The listing builds one solid part. Answer for the finished solid, in the listing's coordinates (mm). Face numbers are marked on the shaded views. A direction names the side the tool comes from. Coordinates: 2 decimals unless noted, no trailing zeros. Write each loop counter-clockwise with the first axis right and the second up, starting at its lowest first coordinate (ties: lowest second). Pieces come first, ordered by that corner, then holes.
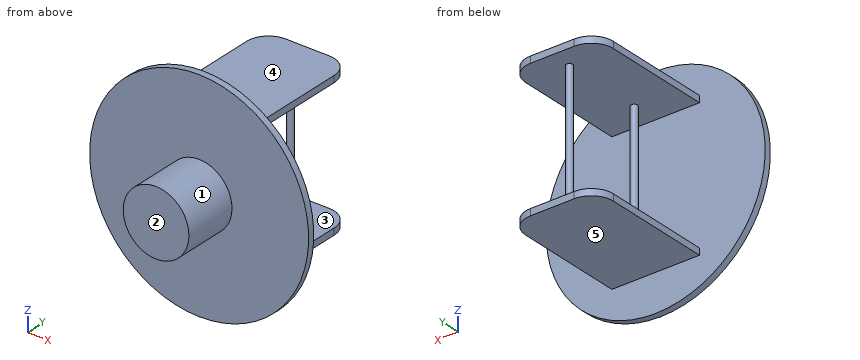
from build123d import *

# Parameters (mm, degrees)
SKETCH1_R           = 50
BOSS_EXTRUDE1_DEPTH = 3
SKETCH2_R           = 15
BOSS_EXTRUDE2_DEPTH = 25
SKETCH3_W           = 40
SKETCH3_H           = 3
BOSS_EXTRUDE3_DEPTH = 60
SKETCH4_R           = 1.5
BOSS_EXTRUDE4_DEPTH = 63
FILLET1_R           = 10


with BuildPart() as part:
    # Sketch1 → Boss-Extrude1 (new body)
    with BuildSketch(Plane(origin=(0, 0, 0), x_dir=(1, 0, 0), z_dir=(0, 1, 0))):
        with Locations(Location((0, 0, 0), (0, 0, 270))):
            Circle(SKETCH1_R)
    extrude(amount=BOSS_EXTRUDE1_DEPTH)

    # Sketch2 → Boss-Extrude2 (add)
    with BuildSketch(Plane(origin=(0, 0, 0), x_dir=(-1, 0, 0), z_dir=(0, -1, 0))):
        with Locations(Location((0, 0, 0), (0, 0, 90))):
            Circle(SKETCH2_R)
    extrude(amount=BOSS_EXTRUDE2_DEPTH)

    # Sketch3 → Boss-Extrude3 (add)
    with BuildSketch(Plane(origin=(0, 3, 0), x_dir=(1, 0, 0), z_dir=(0, 1, 0))):
        with Locations((0, -31.5)):
            Rectangle(SKETCH3_W, SKETCH3_H)
        with Locations((0, 31.5)):
            Rectangle(SKETCH3_W, SKETCH3_H)
    extrude(amount=BOSS_EXTRUDE3_DEPTH)

    # Sketch4 → Boss-Extrude4 (add)
    with BuildSketch(Plane.XY.offset(33)):
        with Locations((0, 53)):
            Circle(SKETCH4_R)
        with Locations((0, 15.5)):
            Circle(SKETCH4_R)
    extrude(amount=-BOSS_EXTRUDE4_DEPTH)

    # Fillet1
    fillet1_edges = [part.edges().sort_by_distance(p)[0] for p in [
        (-20, 63, 31.5),
        (20, 63, 31.5),
        (-20, 63, -31.5),
        (20, 63, -31.5),
    ]]
    fillet(fillet1_edges, radius=FILLET1_R)


solid = part.part
Q1. The part is cut by section C-C, the plane x = 0. Write down the section's boundary in (y, z), then the cut area to 3 significant figures.
Answers below:
outline: (-25, -15) - (0, -15) - (0, -50) - (3, -50) - (3, -33) - (63, -33) - (63, -30) - (54.5, -30) - (54.5, 30) - (63, 30) - (63, 33) - (3, 33) - (3, 50) - (0, 50) - (0, 15) - (-25, 15) - close; hole (3, -30) - (14, -30) - (14, 30) - (3, 30) - close; hole (17, -30) - (51.5, -30) - (51.5, 30) - (17, 30) - close
area: 1,770 mm2
Q2. Determine the mould class of the marked faces 3, 4 and 5 for opening direction Z: released by +Z, released by -Z, zero draft, split by the parting line, or undercut.
Answers below:
face 3: undercut
face 4: released by +Z
face 5: released by -Z
Q3. Which of the six approach directions +Z, -Z, +X, -X, +Y, -Y give full straight-line access (tool end or side, diameter ignored) to the marked faces 1 and 2?
Answers below:
face 1: -Y
face 2: +Z, -Z, +X, -X, -Y
Q4. Find the intervals of material crossed by probe 1 along Z at (x, y) = (-14, 45); probe 2 along Y at (x, z) = (-27, -27.5); probe 3 along Y at (x, z) = (8.5, 12), in increasing order.
Answers below:
probe 1: z = -33 to -30, 30 to 33
probe 2: y = 0 to 3
probe 3: y = -25 to 3
Q5. The part is cut by section A-A, the plane y = 42. Write down the section's boundary in (x, z).
Answers below:
outline: (-20, -33) - (20, -33) - (20, -30) - (-20, -30) - close; (-20, 30) - (20, 30) - (20, 33) - (-20, 33) - close
Q6. The part is cut by section B-B, the plane z = 0. Write down the section's boundary in (x, y), then the cut area to 3 significant figures.
Answers below:
outline: (-50, 0) - (-15, 0) - (-15, -25) - (15, -25) - (15, 0) - (50, 0) - (50, 3) - (-50, 3) - close; circle Ø3 at (0, 15.5); circle Ø3 at (0, 53)
area: 1,060 mm2
Q7. The part is cut by section D-D, the plane y = 15.5. Write down the section's boundary in (x, z), then the cut area to 3 significant figures.
Answers below:
outline: (-20, -33) - (20, -33) - (20, -30) - (1.5, -30) - (1.5, 30) - (20, 30) - (20, 33) - (-20, 33) - (-20, 30) - (-1.5, 30) - (-1.5, -30) - (-20, -30) - close
area: 420 mm2
Q8. Given pin 1 (3.5 mm diameter, centred on y = 37.5, z = -32, fed in from -X); pin 2 (1.5 mm diameter, centred on x = 0.5, z = 14, fed in from +Y); pin 3 (4 mm diameter, centred on x = -38.5, z = -29, fed in from +Y), each flat-ended and moving along its own axis, determine where each tip first touches the part or whether it passes through.
Answers below:
pin 1: stops at x = -20
pin 2: stops at y = 54.5
pin 3: stops at y = 3
